Can you work these out from the model? Positions are in its coordinate system, mm. A direction names the side the tool comes from. Coordinates: 2 decimals unless noted, no trailing zeros. Loops run counter-clockwise (first coordinate to the right, second up) from the corner with the lowest first, then second, coordinate; pieces in that order, holes last. Notation, with made-up numbers: M -1,-2.75 L 47,-2.75 A19 ccw 47,3.25 Z; hole C -15,45 d8. An arc over 180 degrees is marked long. Answer as a JSON object with one key per item and string values. Group by question number.
Item 1: If I drill on line 1 (Y direction, x = 25.4, z = -7) (3 decimals); line 2 (Y direction, x = -25.4, z = -14.75) (3 decimals); line 3 (Y direction, x = 9, z = -29), over which ranges is the centre line in solid material (lowest first)?
Item 2: I'm going to push flat-ended pins straight in: pin 1 Ø1 at (x, y) = (11.5, 19) entering from -Z; pin 2 Ø6 at (x, y) = (-25.4, 6.35) entering from -Z; pin 3 Ø6.5 at (x, y) = (-25, 8) entering from -Z; pin 4 Ø8 at (x, y) = (-25.4, 28.575) entering from +Z. Where does each tip first touch, or does it pass through?
Item 3: Suppose I cut it at C-C (y = 11.5). Write out the boundary of the cut face in (x, z).
Item 4: Suppose I cut it at D-D (y = 29.5). Write out the boundary of the cut face in (x, z), then the cut area to 3 significant figures.
Item 5: Suppose I cut it at A-A (y = 6.35). Count the separate pieces of the cut face and the enclosed holes in it, then the cut area to 3 significant figures.
Item 6: We'd pull the mould along X, two halves only. Please class faces 3 (the cylindrical face through (-0.676, 17.24, -31.743)), 4 (the cylindrical face through (-20.958, 6.509, -17.116)), 5 (the flat face through (25, 18, -1.588)): +X half, -X half, draft (parallel to the pull), parting line (faces both ways), or undercut.
Item 7: Which directions (+Z, -Z, +X, -X, +Y, -Y) give clear straight access to the entire face, cutting with the end or side of a thin tool? Please do faces 1 (the flat face through (0.4, 0, -19.3)), 2 (the flat face through (23, 27, -12.7)).
```python
from build123d import *

# Parameters (mm, degrees)
BOSS_EXTRUDE1_DEPTH        = 34.925
F_8_0_199_DIAMETER_HOLE1_D = 5.0546
LPATTERN1_COUNT            = 2
LPATTERN1_PITCH            = 50.8
LPATTERN1_COUNT_DIR2       = 2
LPATTERN1_PITCH_DIR2       = 22.225
SKETCH5_R                  = 4.445
CUT_EXTRUDE1_DEPTH         = 19.05
LPATTERN2_COUNT            = 2
LPATTERN2_PITCH            = 50.8
LPATTERN2_COUNT_DIR2       = 2
LPATTERN2_PITCH_DIR2       = 22.225
FILLET1_R                  = 1.5875
SKETCH6_W                  = 63.605048243
SKETCH6_H                  = 35.055385684
CUT_EXTRUDE3_DEPTH         = 1.5875


with BuildPart() as part:
    # Sketch1 → Boss-Extrude1 (new body)
    with BuildSketch(Plane(origin=(0, 0, 0), x_dir=(1, 0, 0), z_dir=(0, 1, 0))):
        with BuildLine():
            Line((-19.05, 0), (-31.75, 0))
            ThreePointArc((-31.75, 0), (0, 31.75), (31.75, 0))
            Line((31.75, 0), (19.05, 0))
            ThreePointArc((19.05, 0), (0, 19.05), (-19.05, 0))
        make_face()
    extrude(amount=BOSS_EXTRUDE1_DEPTH)

    # #8 (0.199) Diameter Hole1 (through all)
    with Locations(Plane.XY):
        with Locations((-25.4, 28.575)):
            f_8_0_199_diameter_hole1 = Hole(F_8_0_199_DIAMETER_HOLE1_D / 2)

    # LPattern1: 8 _0.199_ Diameter Hole1 2 × 2
    with Locations(*[(i * LPATTERN1_PITCH, -j * LPATTERN1_PITCH_DIR2, 0) for i in range(LPATTERN1_COUNT) for j in range(LPATTERN1_COUNT_DIR2) if (i, j) != (0, 0)]):
        add(f_8_0_199_diameter_hole1, mode=Mode.SUBTRACT)

    # Sketch5 → Cut-Extrude1 (cut)
    with BuildSketch(Plane(origin=(0, 0, -31.75), x_dir=(-1, 0, 0), z_dir=(0, 0, -1))):
        with Locations((-25.4, 28.575)):
            Circle(SKETCH5_R)
    cut_extrude1 = extrude(amount=-CUT_EXTRUDE1_DEPTH, mode=Mode.SUBTRACT)

    # LPattern2: Cut-Extrude1 2 × 2
    with Locations(*[(-i * LPATTERN2_PITCH, -j * LPATTERN2_PITCH_DIR2, 0) for i in range(LPATTERN2_COUNT) for j in range(LPATTERN2_COUNT_DIR2) if (i, j) != (0, 0)]):
        add(cut_extrude1, mode=Mode.SUBTRACT)

    # Fillet1
    fillet1_edges = [part.edges().sort_by_distance(p)[0] for p in [
        (0, 34.925, -31.75),
        (0, 0, -31.75),
    ]]
    fillet(fillet1_edges, radius=FILLET1_R)

    # Sketch6 → Cut-Extrude3 (cut)
    with BuildSketch(Plane(origin=(0, 0, 0), x_dir=(-1, 0, 0), z_dir=(0, 0, -1))):
        with Locations((0.052524121, 17.397307158)):
            Rectangle(SKETCH6_W, SKETCH6_H)
    extrude(amount=CUT_EXTRUDE3_DEPTH, mode=Mode.SUBTRACT)


solid = part.part
```
From the geometry:
{
 "1": {"line 1": "0 to 3.823, 8.877 to 26.048, 31.102 to 34.925", "line 2": "0 to 1.905, 10.795 to 24.13, 33.02 to 34.925", "line 3": "0.01 to 34.91"},
 "2": {"pin 1": "z = -29.78", "pin 2": "z = -12.7", "pin 3": "z = -22.92", "pin 4": "z = -1.59"},
 "3": {"outline": "M -31.71,-1.59 A31.75 ccw 31.71,-1.59 L 18.98,-1.59 A19.05 cw -18.98,-1.59 Z"},
 "4": {"outline": "M -31.71,-1.59 A31.75 ccw -29.1,-12.7 L -27.75,-12.7 L -27.75,-1.59 Z; M -23.05,-12.7 L -21.05,-12.7 L -21.05,-23.77 A31.75 ccw 21.05,-23.77 L 21.05,-12.7 L 23.05,-12.7 L 23.05,-1.59 L 18.98,-1.59 A19.05 cw -18.98,-1.59 L -23.05,-1.59 Z; M 27.75,-12.7 L 29.1,-12.7 A31.75 ccw 31.71,-1.59 L 27.75,-1.59 Z", "area": "766 mm2"},
 "5": {"separate pieces": "3", "enclosed holes": "0", "area": "756 mm2"},
 "6": {"face 3": "parting line", "face 4": "undercut", "face 5": "draft"},
 "7": {"face 1": "+Z, -Z, +X, -X, -Y", "face 2": "-Z"}
}
